Work out the finished part from the listing and answer in its coordinate system (mm). Face numbers are marked on the shaded views. A direction names the side the tool comes from. Round coordinates to 2 decimals unless told otherwise and drop trailing zeros. Loops run counter-clockwise (first coordinate to the right, second up) from the corner with the lowest first, then second, coordinate; pieces in that order, holes last.
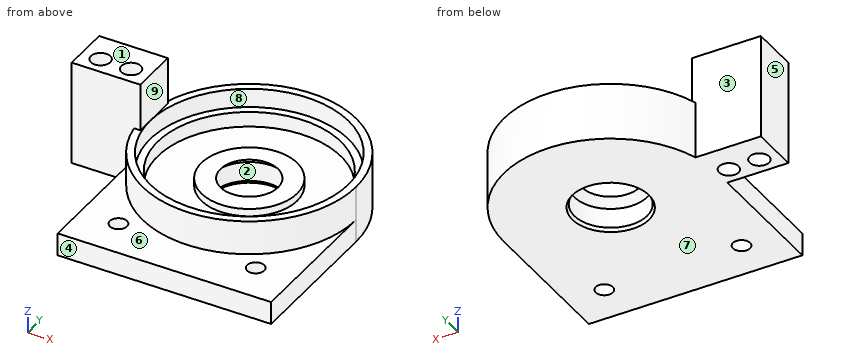
from build123d import *

# Parameters (mm, degrees)
SKETCH040_R   = 28
SKETCH040_R_2 = 9.55
PAD025_DEPTH  = 6
SKETCH038_R   = 28
SKETCH038_R_2 = 26
PAD023_DEPTH  = 15
SKETCH039_R   = 2.25
PAD024_DEPTH  = 6
SKETCH091_R   = 28
SKETCH091_R_2 = 24
PAD056_DEPTH  = 10
SKETCH098_W   = 18
SKETCH098_H   = 12.5
SKETCH098_R   = 2.55
PAD060_DEPTH  = 27.5


with BuildPart() as part:
    # Sketch040 → Pad025 (new body)
    with BuildSketch(Plane.XY):
        Circle(SKETCH040_R)
        Circle(SKETCH040_R_2, mode=Mode.SUBTRACT)
    extrude(amount=PAD025_DEPTH)

    # Sketch038 → Pad023 (join)
    with BuildSketch(Plane.XY):
        Circle(SKETCH038_R)
        Circle(SKETCH038_R_2, mode=Mode.SUBTRACT)
    extrude(amount=PAD023_DEPTH)

    # Sketch039 → Pad024 (join)
    with BuildSketch(Plane.XY):
        with BuildLine():
            ThreePointArc((-28, 0), (0, -28), (28, 0))
            Line((28, -38.6375), (28, 0))
            Line((-28, -38.6375), (28, -38.6375))
            Line((-28, 0), (-28, -38.6375))
        make_face()
        with Locations((-18, -28.31875)):
            Circle(SKETCH039_R, mode=Mode.SUBTRACT)
        with Locations((18, -28.31875)):
            Circle(SKETCH039_R, mode=Mode.SUBTRACT)
    extrude(amount=PAD024_DEPTH)

    # Sketch041 → Groove (revolve, cut)
    with BuildSketch(Plane.YZ):
        Polygon((9.55, 0.866025), (10.05, 0), (9.55, 0), align=None)
    revolve(axis=Axis((0, 0, 0), (0, 0, 1)), mode=Mode.SUBTRACT)

    # Sketch065 → Revolution (revolve)
    with BuildSketch(Plane.XZ):
        Polygon((9.55, 6), (7.55, 8), (12.55, 8), (12.55, 6), align=None)
    revolve(axis=Axis((0, 0, 0), (0, 0, 1)))

    # Sketch091 → Pad056 (join)
    with BuildSketch(Plane.XY):
        Circle(SKETCH091_R)
        Circle(SKETCH091_R_2, mode=Mode.SUBTRACT)
    extrude(amount=PAD056_DEPTH)

    # Sketch098 → Pad060 (join)
    with BuildSketch(Plane.XY):
        with Locations((-35, 1.75)):
            Rectangle(SKETCH098_W, SKETCH098_H)
        with Locations((-39, 0)):
            Circle(SKETCH098_R, mode=Mode.SUBTRACT)
        with Locations((-31, 0)):
            Circle(SKETCH098_R, mode=Mode.SUBTRACT)
    extrude(amount=PAD060_DEPTH)


solid = part.part
Item 1: Straight lines are drawn through the part: line 1 (Y direction, x = 1, z = 14); line 2 (Z direction, x = 21, y = -20); line 3 (Y direction, x = -35.5, z = 8.25). For each, find the intervals that lie inside material, in ascending order.
Item 2: Section A-A, the plane x = 0 is taken. Give the vertices of the cut face in (y, z), plus the area to 3 significant figures.
Item 3: Determine the mould class of the marked faces 1, 2, 3 and 4 for opening direction Y: pulls with the +Y half, pulls with the -Y half, needs draft (parallel to the pull), parting line crosses it, or undercut.
Item 4: Each of these flat-tipped pins is pushed along its axis until it touches: P1, Ø3, axis at x = -8.5, z = 15, coming from the +Y side; P2, Ø6.5, axis at y = -27.5, z = 2.5, coming from the -X side; P3, Ø24, axis at x = -3, y = 9, coming from the +Z side. Where does it stop, or does it pass through?
Item 5: For the marked faces 5, 6, 7, 8 and 9, determine the directions among +Z, -Z, +X, -X, +Y, -Y from which every point of the face is accessible in a straight line to the end or side of a thin tool.
Item 6: Section D-D, the plane x = -39 is taken. Give the vertices of the cut face in (y, z).
Item 7: Section B-B, the plane z = 9 is taken. Give the vertices of the cut face in (x, y), plus the area to 3 significant figures.
Item 8: Section C-C, the plane z = 25.25 is taken. Give the vertices of the cut face in (x, y).
Answer below:
1. line 1: y = -27.98 to -25.98, 25.98 to 27.98
1. line 2: z = 0 to 6
1. line 3: y = -4.5 to 8
2. outline: (-38.64, 0) - (-10.05, 0) - (-9.55, 0.87) - (-9.55, 6) - (-7.55, 8) - (-12.55, 8) - (-12.55, 6) - (-24, 6) - (-24, 10) - (-26, 10) - (-26, 15) - (-28, 15) - (-28, 6) - (-38.64, 6) - close; (7.55, 8) - (9.55, 6) - (9.55, 0.87) - (10.05, 0) - (28, 0) - (28, 15) - (26, 15) - (26, 10) - (24, 10) - (24, 6) - (12.55, 6) - (12.55, 8) - close
2. area: 353 mm2
3. face 1: needs draft
3. face 2: undercut
3. face 3: pulls with the +Y half
3. face 4: pulls with the -Y half
4. P1: stops at y = 27.11
4. P2: stops at x = -28
4. P3: stops at z = 8
5. face 5: +Z, -Z, -X, +Y, -Y
5. face 6: +Z, -Y
5. face 7: -Z, +X, -X, +Y, -Y
5. face 8: +Z
5. face 9: +Z, +X, +Y, -Y
6. outline: (-4.5, 0) - (-2.55, 0) - (-2.55, 27.5) - (-4.5, 27.5) - close; (2.55, 0) - (8, 0) - (8, 27.5) - (2.55, 27.5) - close
7. outline: (-44, -4.5) - (-27.64, -4.5) arc R28 ccw (long way) to (-26.83, 8) - (-44, 8) - close; hole circle Ø5.1 at (-39, 0); hole circle Ø5.1 at (-31, 0); hole circle Ø48 at (0, 0)
7. area: 816 mm2
8. outline: (-44, -4.5) - (-26, -4.5) - (-26, 8) - (-44, 8) - close; hole circle Ø5.1 at (-39, 0); hole circle Ø5.1 at (-31, 0)
